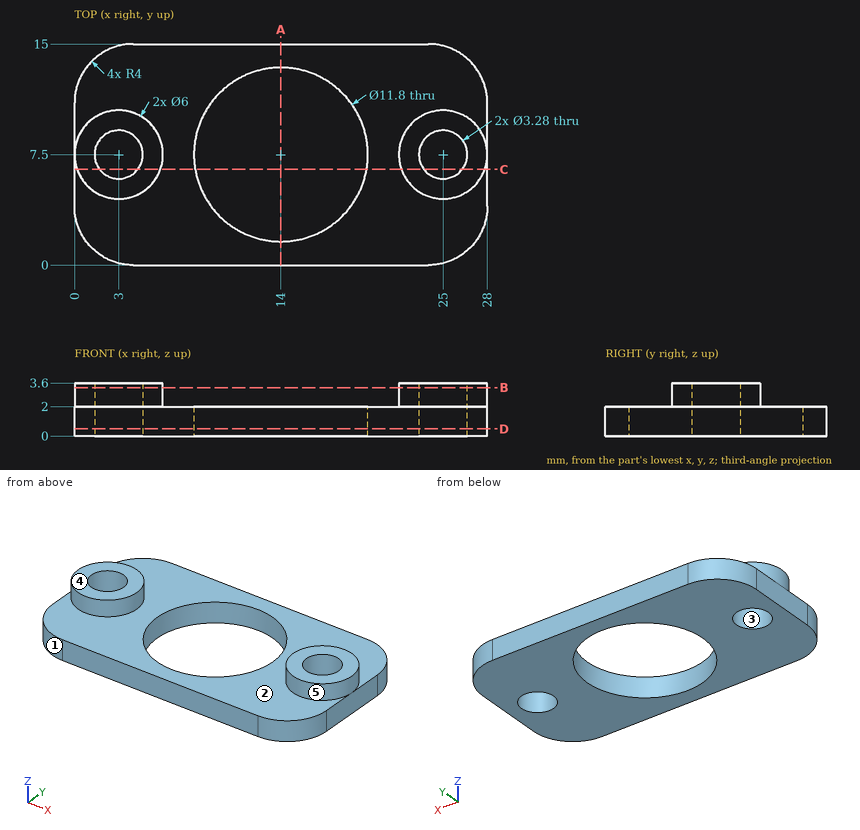
Part print with two shaded views. Sizes in mm from the minimum x, y, z corner. A direction names the side the tool comes from. Round coordinates to 2 decimals unless told otherwise and drop trailing zeros. Order: outer loops, then holes, each group sorted by start corner. A loop starts at its lowest first (then second) coordinate and runs counter-clockwise, first axis right, second up.
(1) Band-saw the part on C-C (y = 6.5). List the corners of the cut face in (x, z).
(2) Drill centre lines: line 1 (Y direction, x = 25, z = 2.35); line 2 (X direction, y = 6.75, z = 1.8); line 3 (X direction, y = 6, z = 0.65). Where is each one in solid material? Low to high.
(3) 3-axis set-ups, long thin cutter, end or side, ignore diameter. For the marked faces 1 and 2: which of +Z, -Z, +X, -X, +Y, -Y reach the whole face in a straight line?
(4) Pin check, flat tip, straight feed: pin 1 (3 mm diameter, centred on x = 4, y = 3.5, fed in from +Z). Stop position of the tip, or through.
(5) Pull direction Y, two halves, no side cores. Call the marked faces 3, 4 and 5: released by +Y, released by -Y, zero draft, split by the parting line, or undercut.
(6) Band-saw the part on A-A (x = 14). List the corners of the cut face in (y, z), then the cut area to 3 significant figures.
(7) Band-saw the part on B-B (z = 3.3). List the corners of the cut face in (x, y), then the cut area to 3 significant figures.
(8) Band-saw the part on D-D (z = 0.5). List the corners of the cut face in (x, y).
Verdict:
1. outline: (0, 0) - (1.7, 0) - (1.7, 3.6) - (0.17, 3.6) - (0.17, 2) - (0, 2) - close; (4.3, 0) - (8.19, 0) - (8.19, 2) - (5.83, 2) - (5.83, 3.6) - (4.3, 3.6) - close; (19.81, 0) - (23.7, 0) - (23.7, 3.6) - (22.17, 3.6) - (22.17, 2) - (19.81, 2) - close; (26.3, 0) - (28, 0) - (28, 2) - (27.83, 2) - (27.83, 3.6) - (26.3, 3.6) - close
2. line 1: y = 4.5 to 5.86, 9.14 to 10.5
2. line 2: x = 0 to 1.54, 4.46 to 8.15, 19.85 to 23.54, 26.46 to 28
2. line 3: x = 0 to 2.34, 3.66 to 8.29, 19.71 to 24.34, 25.66 to 28
3. face 1: +Z, -Z, -X, -Y
3. face 2: +Z
4. pin 1: stops at z = 3.6
5. face 3: undercut
5. face 4: zero draft
5. face 5: split by the parting line
6. outline: (0, 0) - (1.6, 0) - (1.6, 2) - (0, 2) - close; (13.4, 0) - (15, 0) - (15, 2) - (13.4, 2) - close
6. area: 6.40 mm2
7. outline: circle Ø6 at (3, 7.5); circle Ø6 at (25, 7.5); hole circle Ø3.28 at (3, 7.5); hole circle Ø3.28 at (25, 7.5)
7. area: 39.6 mm2
8. outline: (0, 4) arc R4 ccw to (4, 0) - (24, 0) arc R4 ccw to (28, 4) - (28, 11) arc R4 ccw to (24, 15) - (4, 15) arc R4 ccw to (0, 11) - close; hole circle Ø3.28 at (3, 7.5); hole circle Ø11.8 at (14, 7.5); hole circle Ø3.28 at (25, 7.5)
